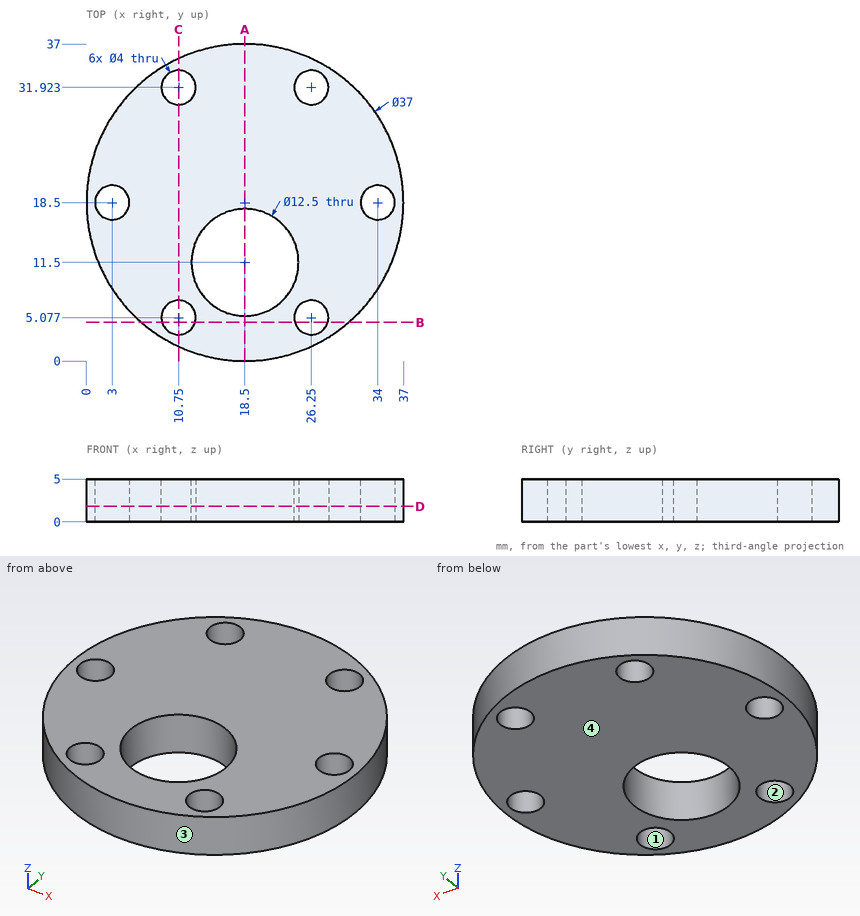
Geometry check sheet. Reference: drawing and pictorial views, mm from the part's lowest x, y, z. Round coordinates to 2 decimals unless told otherwise and drop trailing zeros. Loops run counter-clockwise (first coordinate to the right, second up) from the corner with the lowest first, then second, coordinate; pieces in that order, holes last. Notation, with made-up numbers: (26, 35.25) - (72, 35.25) arc R31 cw to (72, 67.25) - close; hole circle Ø6 at (39.25, 1). An arc over 180 degrees is marked (long way). Answer as CSV lines item,"result".
(1) Cross-section at C-C, the plane x = 10.75. Enter the section's corners in (y, z), and give its area (3 significant figures).
Output values:
outline,"(1.7, 0) - (3.08, 0) - (3.08, 5) - (1.7, 5) - close; (7.08, 0) - (29.92, 0) - (29.92, 5) - (7.08, 5) - close; (33.92, 0) - (35.3, 0) - (35.3, 5) - (33.92, 5) - close"
area,"128 mm²"
(2) Depth check by flat-ended pin: pin 1 Ø3.5 at (x, y) = (10.75, 31.92) entering from +Z; pin 2 Ø2 at (x, z) = (12.5, 2.5) entering from -Y. Enter the tip coordinate at first touch or a pass-through.
Output values:
pin 1,"passes through"
pin 2,"stops at y = 0.69"
(3) Material ranges on line 1 along X through (y, z) = (20, 1.5) (1 decimal); line 2 along X through (y, z) = (19.5, 1.95); line 3 along Y through (x, z) = (15.5, 2.85) (1 decimal), recorded low to high.
Output values:
line 1,"x = 0.1 to 1.7, 4.3 to 32.7, 35.3 to 36.9"
line 2,"x = 0.03 to 1.27, 4.73 to 32.27, 35.73 to 36.97"
line 3,"y = 0.2 to 6, 17 to 36.8"
(4) Cross-section at B-B, the plane y = 4.5. Enter the section's corners in (x, z) (1 decimal).
Output values:
outline,"(6.4, 0) - (8.8, 0) - (8.8, 5) - (6.4, 5) - close; (12.7, 0) - (24.3, 0) - (24.3, 5) - (12.7, 5) - close; (28.2, 0) - (30.6, 0) - (30.6, 5) - (28.2, 5) - close"
(5) Cross-section at A-A, the plane x = 18.5. Enter the section's corners in (y, z).
Output values:
outline,"(0, 0) - (5.25, 0) - (5.25, 5) - (0, 5) - close; (17.75, 0) - (37, 0) - (37, 5) - (17.75, 5) - close"
(6) Cross-section at D-D, the plane z = 1.8. Enter the section's corners in (x, y), and give its area (3 significant figures).
Output values:
outline,"circle Ø37 at (18.5, 18.5); hole circle Ø4 at (3, 18.5); hole circle Ø4 at (10.75, 5.08); hole circle Ø4 at (10.75, 31.92); hole circle Ø12.5 at (18.5, 11.5); hole circle Ø4 at (26.25, 5.08); hole circle Ø4 at (26.25, 31.92); hole circle Ø4 at (34, 18.5)"
area,"877 mm²"
(7) Release check for a two-part mould opening along X. For the marked faces 1, 2, 3 and 4 record: released by +X, released by -X, zero draft, split by the parting line, or undercut.
Output values:
face 1,"undercut"
face 2,"undercut"
face 3,"split by the parting line"
face 4,"zero draft"
